Check sheet for the modelled part. Datum: model origin and axes. Units: mm. Coordinates: 2 decimals unless noted, no trailing zeros. Loops run counter-clockwise (first coordinate to the right, second up) from the corner with the lowest first, then second, coordinate; pieces in that order, holes last. Notation, with made-up numbers: (82.5, -31) -> (138.5, -31) arc R20 cw to (138.5, 0) -> close; hole circle Ø8 at (40.25, 2). An arc over 180 degrees is marked (long way). Use CSV: the item, a comma, the result in double quotes. Start each with the question number.
1. Sectioned sample at A-A, the plane x = -139.7. Record the cut outline in (y, z) (1 decimal).
2. Thickness scan on L1, parallel to Z at x = 136.5, y = 0.6; L2, parallel to X at y = 0.85, z = -133.5; L3, parallel to X at y = 0.3, z = 2. Record the ranges inside material, lowest first.
3. Sectioned sample at D-D, the plane z = 182. Record the cut outline in (x, y).
4. Gauge pin test, flat ends, axial feed: pin 1 (0.8 mm diameter, centred on y = 0.5, z = -216.5, fed in from -X); pin 2 (0.5 mm diameter, centred on y = 1, z = 215.5, fed in from -X); pin 3 (1.5 mm diameter, centred on x = -147, z = -81.5, fed in from -Y); pin 4 (0.8 mm diameter, centred on x = 215, y = 0.5, fed in from +Z). Record the tip position at first contact, or that the pin passes through.
5. Sectioned sample at C-C, the plane x = 52.5. Record the cut outline in (y, z).
6. Sectioned sample at B-B, the plane z = 94. Record the cut outline in (x, y), and give its area (3 significant figures).
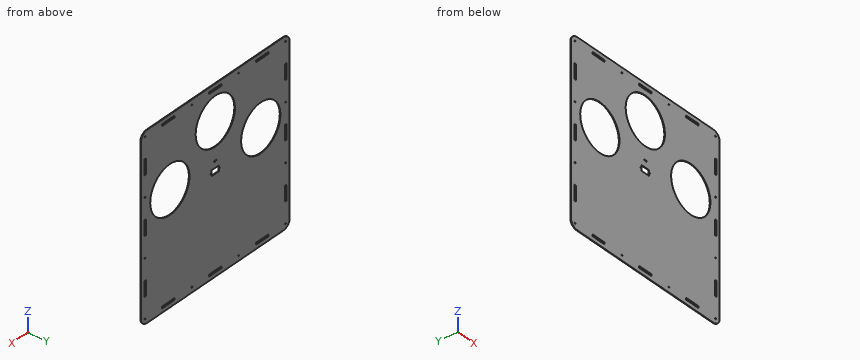
```python
from build123d import *

# Parameters (mm, degrees)
SKETCH1_W             = 457.2
SKETCH1_H             = 457.2
MAIN_PLATE_DEPTH      = 1.5875
SKETCH2_R             = 60.325
DRUM_HOLES_DEPTH      = 1.5875
SKETCH4_R             = 1.190625
SKETCH4_R_2           = 1.5875
IR_HOLES_DEPTH        = 1.5875
SKETCH5_R             = 1.48828125
BOLT_HOLES_DEPTH      = 1.5875
SKETCH7_R             = 1.190625
SKETCH7_W             = 22.86
SKETCH7_H             = 13.97
SERVO_DEPTH           = 1.5875
SKETCH8_W             = 4.7625
SKETCH8_H             = 38.1
SKETCH8_W_2           = 38.1
SKETCH8_H_2           = 4.7625
ALIGNMENT_HOLES_DEPTH = 1.5875
FILLET1_R             = 19.05


with BuildPart() as part:
    # Sketch1 → Main Plate (new body)
    with BuildSketch(Plane(origin=(0, 0, 0), x_dir=(1, 0, 0), z_dir=(0, 1, 0))):
        Rectangle(SKETCH1_W, SKETCH1_H)
    extrude(amount=MAIN_PLATE_DEPTH)

    # Sketch2 → Drum Holes (cut)
    with BuildSketch(Plane(origin=(0, 1.5875, 0), x_dir=(1, 0, 0), z_dir=(0, 1, 0))):
        with Locations(Location((0, -139.7, 0), (0, 0, 270))):
            Circle(SKETCH2_R)
        with Locations(Location((-139.7, -50.8, 0), (0, 0, 270))):
            Circle(SKETCH2_R)
        with Locations(Location((139.7, -50.8, 0), (0, 0, 90))):
            Circle(SKETCH2_R)
    extrude(amount=-DRUM_HOLES_DEPTH, mode=Mode.SUBTRACT)

    # Sketch4 → IR Holes (cut)
    with BuildSketch(Plane(origin=(0, 1.5875, 0), x_dir=(1, 0, 0), z_dir=(0, 1, 0))):
        with Locations(Location((-2.38125, -45.72, 0), (0, 0, 270))):
            Circle(SKETCH4_R)
        with Locations(Location((2.38125, -45.72, 0), (0, 0, 270))):
            Circle(SKETCH4_R_2)
    extrude(amount=-IR_HOLES_DEPTH, mode=Mode.SUBTRACT)

    # Sketch5 → Bolt Holes (cut)
    with BuildSketch(Plane(origin=(0, 1.5875, 0), x_dir=(1, 0, 0), z_dir=(0, 1, 0))):
        with Locations(Location((-215.9, 215.9, 0), (0, 0, 270))):
            Circle(SKETCH5_R)
        with Locations(Location((-215.9, 71.966666667, 0), (0, 0, 270))):
            Circle(SKETCH5_R)
        with Locations(Location((-215.9, -71.966666667, 0), (0, 0, 270))):
            Circle(SKETCH5_R)
        with Locations(Location((-215.9, -215.9, 0), (0, 0, 270))):
            Circle(SKETCH5_R)
        with Locations(Location((-71.882, 215.9, 0), (0, 0, 270))):
            Circle(SKETCH5_R)
        with Locations(Location((72.136, 215.9, 0), (0, 0, 270))):
            Circle(SKETCH5_R)
        with Locations(Location((215.9, 215.9, 0), (0, 0, 90))):
            Circle(SKETCH5_R)
        with Locations(Location((215.9, 71.966666667, 0), (0, 0, 90))):
            Circle(SKETCH5_R)
        with Locations(Location((215.9, -71.966666667, 0), (0, 0, 90))):
            Circle(SKETCH5_R)
        with Locations(Location((215.9, -215.9, 0), (0, 0, 90))):
            Circle(SKETCH5_R)
        with Locations(Location((72.136, -215.9, 0), (0, 0, 90))):
            Circle(SKETCH5_R)
        with Locations(Location((-71.882, -215.9, 0), (0, 0, 90))):
            Circle(SKETCH5_R)
    extrude(amount=-BOLT_HOLES_DEPTH, mode=Mode.SUBTRACT)

    # Sketch7 → Servo (cut)
    with BuildSketch(Plane(origin=(0, 1.5875, 0), x_dir=(1, 0, 0), z_dir=(0, 1, 0))):
        with Locations(Location((-13.890625, -22.225, 0), (0, 0, 270))):
            Circle(SKETCH7_R)
        with Locations(Location((13.890625, -22.225, 0), (0, 0, 270))):
            Circle(SKETCH7_R)
        with Locations((0, -22.225)):
            Rectangle(SKETCH7_W, SKETCH7_H)
    extrude(amount=-SERVO_DEPTH, mode=Mode.SUBTRACT)

    # Sketch8 → Alignment Holes (cut)
    with BuildSketch(Plane(origin=(0, 1.5875, 0), x_dir=(1, 0, 0), z_dir=(0, 1, 0))):
        with Locations((-215.9, -143.933333333)):
            Rectangle(SKETCH8_W, SKETCH8_H)
        with Locations((-215.9, 0)):
            Rectangle(SKETCH8_W, SKETCH8_H)
        with Locations((215.9, -143.933333333)):
            Rectangle(SKETCH8_W, SKETCH8_H)
        with Locations((-215.9, 143.933333333)):
            Rectangle(SKETCH8_W, SKETCH8_H)
        with Locations((215.9, 0)):
            Rectangle(SKETCH8_W, SKETCH8_H)
        with Locations((215.9, 143.933333333)):
            Rectangle(SKETCH8_W, SKETCH8_H)
        with Locations((-143.891, 215.9)):
            Rectangle(SKETCH8_W_2, SKETCH8_H_2)
        with Locations((144.018, 215.9)):
            Rectangle(SKETCH8_W_2, SKETCH8_H_2)
        with Locations((0, 215.9)):
            Rectangle(SKETCH8_W_2, SKETCH8_H_2)
        with Locations((144.018, -215.9)):
            Rectangle(SKETCH8_W_2, SKETCH8_H_2)
        with Locations((0, -215.9)):
            Rectangle(SKETCH8_W_2, SKETCH8_H_2)
        with Locations((-143.891, -215.9)):
            Rectangle(SKETCH8_W_2, SKETCH8_H_2)
    extrude(amount=-ALIGNMENT_HOLES_DEPTH, mode=Mode.SUBTRACT)

    # Fillet1
    fillet1_edges = [part.edges().sort_by_distance(p)[0] for p in [
        (228.6, 0.79375, 228.6),
        (-228.6, 0.79375, 228.6),
        (-228.6, 0.79375, -228.6),
        (228.6, 0.79375, -228.6),
    ]]
    fillet(fillet1_edges, radius=FILLET1_R)


solid = part.part
```
Completed:
1,outline,"(0, -228.6) -> (1.6, -228.6) -> (1.6, -218.3) -> (0, -218.3) -> close; (0, -213.5) -> (1.6, -213.5) -> (1.6, -9.5) -> (0, -9.5) -> close; (0, 111.1) -> (1.6, 111.1) -> (1.6, 213.5) -> (0, 213.5) -> close; (0, 218.3) -> (1.6, 218.3) -> (1.6, 228.6) -> (0, 228.6) -> close"
2,L1,"-228.6 to -218.28, -213.52 to -9.44, 111.04 to 213.52, 218.28 to 228.6"
2,L2,"-228.6 to -218.28, -213.52 to 213.52, 218.28 to 228.6"
2,L3,"-228.6 to -218.28, -213.52 to -175.16, -104.24 to 104.24, 175.16 to 213.52, 218.28 to 228.6"
3,outline,"(-228.6, 0) -> (-43.01, 0) -> (-43.01, 1.59) -> (-228.6, 1.59) -> close; (43.01, 0) -> (228.6, 0) -> (228.6, 1.59) -> (43.01, 1.59) -> close"
4,pin 1,"x = -227.44"
4,pin 2,"x = -227.73"
4,pin 3,"y = 0"
4,pin 4,"z = 227.92"
5,outline,"(0, -228.6) -> (1.59, -228.6) -> (1.59, 109.99) -> (0, 109.99) -> close; (0, 169.41) -> (1.59, 169.41) -> (1.59, 228.6) -> (0, 228.6) -> close"
6,outline,"(-228.6, 0) -> (-181.81, 0) -> (-181.81, 1.59) -> (-228.6, 1.59) -> close; (-97.59, 0) -> (-39.38, 0) -> (-39.38, 1.59) -> (-97.59, 1.59) -> close; (39.38, 0) -> (97.59, 0) -> (97.59, 1.59) -> (39.38, 1.59) -> close; (181.81, 0) -> (228.6, 0) -> (228.6, 1.59) -> (181.81, 1.59) -> close"
6,area,"333 mm²"
